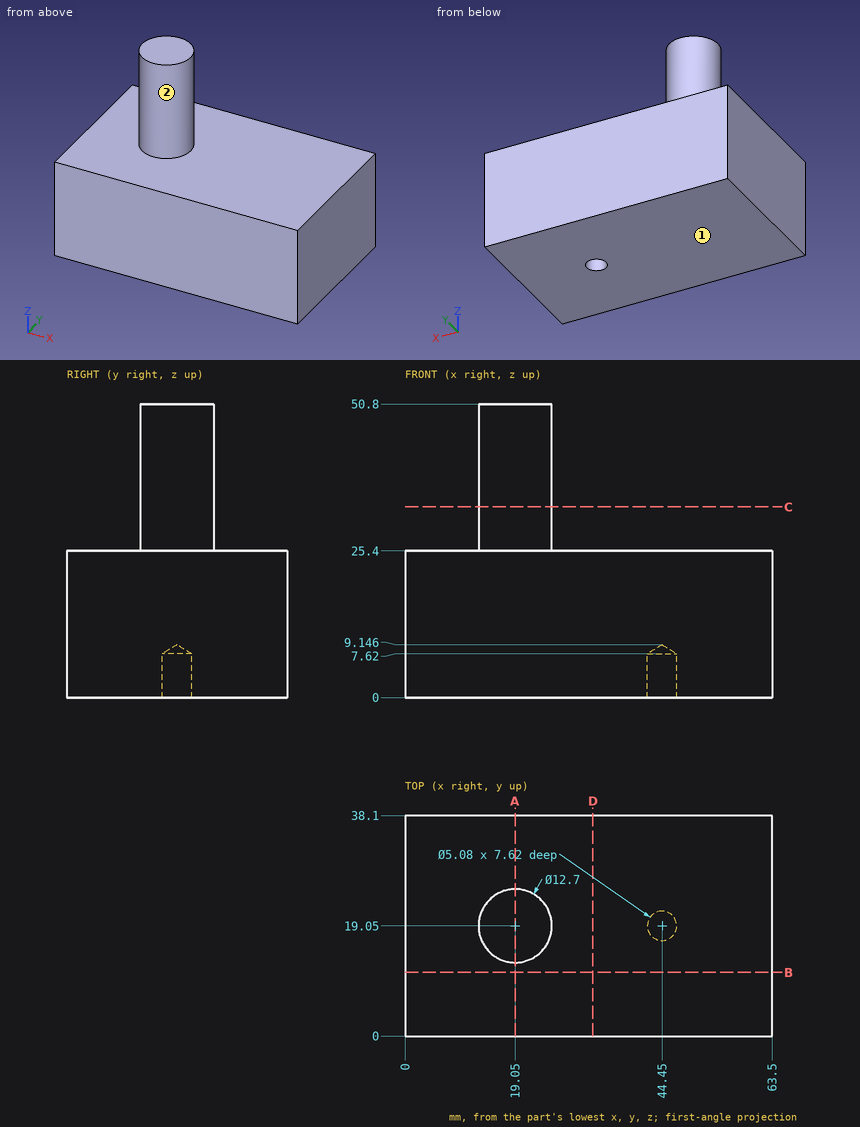
The figure shows three views and two pictorial views of one solid part (mm, origin at its lowest corner). Answer the questions. A direction names the side the tool comes from. Coordinates: 2 decimals unless noted, no trailing zeros. Write each loop counter-clockwise with the first axis right and the second up, starting at its lowest first coordinate (ties: lowest second). Pieces come first, ordered by that corner, then holes. Notation, with made-up numbers: (22, 34.25) -> (35, 34.25) arc R36 ccw to (35, 69.25) -> close; hole circle Ø7 at (-14, 82). An arc over 180 degrees is marked (long way). Answer as a JSON object with one key per item and string values.
Q1. A tool of negligible diameter and unlimited length cuts with its end or side. For the marked faces 1 and 2, from which of +Z, -Z, +X, -X, +Y, -Y can it reach the whole face along a straight path? Write none if from no direction.
The answers:
{"face 1": "-Z, +X, -X, +Y, -Y", "face 2": "+Z"}
Q2. Consider line 1 (X direction, y = 19.05, z = 6); line 2 (Y direction, x = 44.45, z = 2.75); line 3 (Z direction, x = 42, y = 25). Determine where each line is inside the solid, lowest interval first. Write a range as [from, to].
The answers:
{"line 1": "x = [0, 41.91], [46.99, 63.5]", "line 2": "y = [0, 16.51], [21.59, 38.1]", "line 3": "z = [0, 25.4]"}
Q3. Flat-ended cylindrical pins translate along their axes: pin 1 Ø10 at (x, z) = (40, 30) entering from -Y; pin 2 Ø1.5 at (x, y) = (8.5, 34) entering from +Z; pin 3 Ø4 at (x, y) = (44.45, 19.05) entering from -Z (1 decimal); pin 4 Ø3 at (x, z) = (27.5, 35) entering from -Y. Find the tip coordinate at first contact, or state that the pin passes through.
The answers:
{"pin 1": "stops at y = 0", "pin 2": "stops at z = 25.4", "pin 3": "stops at z = 7.9", "pin 4": "passes through"}
Q4. The part is cut by section C-C on z = 33. Give the vertices of the cut face in (x, y), then the cut area to 3 significant figures.
The answers:
{"outline": "circle Ø12.7 at (19.05, 19.05)", "area": "127 mm2"}
Q5. The part is cut by section A-A on x = 19.05. Give the vertices of the cut face in (y, z), then the cut area to 3 significant figures.
The answers:
{"outline": "(0, 0) -> (38.1, 0) -> (38.1, 25.4) -> (25.4, 25.4) -> (25.4, 50.8) -> (12.7, 50.8) -> (12.7, 25.4) -> (0, 25.4) -> close", "area": "1,290 mm2"}
Q6. The part is cut by section B-B on y = 11. Give the vertices of the cut face in (x, z), then the cut area to 3 significant figures.
The answers:
{"outline": "(0, 0) -> (63.5, 0) -> (63.5, 25.4) -> (0, 25.4) -> close", "area": "1,610 mm2"}
Q7. The part is cut by section D-D on x = 32.5. Give the vertices of the cut face in (y, z), then the cut area to 3 significant figures.
The answers:
{"outline": "(0, 0) -> (38.1, 0) -> (38.1, 25.4) -> (0, 25.4) -> close", "area": "968 mm2"}
